Geometry: final body of the model. Coordinates: model frame, mm. A direction names the side the tool comes from. Round coordinates to 2 decimals unless told otherwise and drop trailing zeros. Order: outer loops, then holes, each group sorted by start corner. A loop starts at its lowest first (then second) coordinate and runs counter-clockwise, first axis right, second up. Notation, with made-up numbers: (42.5, -34.5) -> (82.5, -34.5) arc R22 cw to (82.5, -12.5) -> close; hole circle Ø1 at (36.25, 54.25). An arc over 180 degrees is marked (long way). Put each result on its own line as item: value.
```python
from build123d import *

# Parameters (mm, degrees)
SKETCH1_W           = 75
SKETCH1_H           = 75
BOSS_EXTRUDE1_DEPTH = 50
SKETCH2_W           = 71
SKETCH2_H           = 71
CUT_EXTRUDE1_DEPTH  = 48
CUT_EXTRUDE6_DEPTH  = 2
FILLET4_R           = 5
FILLET5_R           = 5
FILLET6_R           = 5
FILLET7_R           = 5
SKETCH4_W           = 10
SKETCH4_H           = 10
BOSS_EXTRUDE2_DEPTH = 44
SKETCH5_W           = 10
SKETCH5_H           = 10
BOSS_EXTRUDE3_DEPTH = 44
SKETCH8_W           = 51
SKETCH8_H           = 1
BOSS_EXTRUDE4_DEPTH = 10
SKETCH9_W           = 51
SKETCH9_H           = 1
BOSS_EXTRUDE5_DEPTH = 10
SKETCH11_R          = 3.25
CUT_EXTRUDE8_DEPTH  = 2.5
SKETCH12_R          = 4.375
CUT_EXTRUDE9_DEPTH  = 2
SKETCH13_R          = 5.838
CUT_EXTRUDE10_DEPTH = 2


with BuildPart() as part:
    # Sketch1 → Boss-Extrude1 (new body)
    with BuildSketch(Plane(origin=(0, 0, 0), x_dir=(1, 0, 0), z_dir=(0, 1, 0))):
        Rectangle(SKETCH1_W, SKETCH1_H)
    extrude(amount=BOSS_EXTRUDE1_DEPTH)

    # Sketch2 → Cut-Extrude1 (cut)
    with BuildSketch(Plane(origin=(0, 50, 0), x_dir=(1, 0, 0), z_dir=(0, 1, 0))):
        Rectangle(SKETCH2_W, SKETCH2_H)
    extrude(amount=-CUT_EXTRUDE1_DEPTH, mode=Mode.SUBTRACT)

    # Sketch3 → Cut-Extrude6 (cut)
    with BuildSketch(Plane.XZ):
        with BuildLine():
            add(Edge.make_bspline(
                [(8.333333333, 0), (8.451740367, 0.002755681), (8.687804992, 0.024362572), (9.156850661, 0.091751534), (10.280456566, 0.34563371), (11.894311549, 0.927153054), (13.898826649, 2.013834871), (16.012913856, 3.730779379), (17.760775609, 5.821518912), (19.049737677, 8.225078468), (19.814659338, 10.889902937), (19.985573746, 13.70225433), (19.539290317, 16.528302053), (18.494901563, 19.237024306), (16.925532574, 21.678165695), (14.89875072, 23.755747946), (12.484340707, 25.370708371), (9.802384445, 26.405476858), (6.98608034, 26.794959186), (4.109785684, 26.53719328), (0.722828385, 25.487699584), (-2.940307765, 23.340193971), (-6.647366, 20.112650151), (-10.3710479, 16.053559605), (-13.910491439, 11.839455496), (-17.496638537, 7.662725627), (-20.98187941, 4.115658379), (-23.987384387, 1.758333025), (-26.330229801, 0.518546697), (-27.55448652, 0.125207567), (-28.000518844, 0.031619583), (-28.254918245, 0.003498461), (-28.299650799, 0.000763354), (-28.322057313, 2.7753e-05), (-28.333267806, 1.08e-07)],
                knots=[0, 0, 0, 0, 0, 0.005562941, 0.011125882, 0.022251763, 0.05405154, 0.085851775, 0.117651832, 0.149451632, 0.181251419, 0.213051359, 0.246907992, 0.280764683, 0.314621503, 0.348478291, 0.382335072, 0.416191783, 0.450048462, 0.482370896, 0.514693479, 0.550840193, 0.615485432, 0.680130557, 0.744775838, 0.809420945, 0.874066354, 0.938711777, 0.978091789, 0.987992515, 0.997893241, 0.998946621, 0.99947331, 1, 1, 1, 1, 1], degree=4))
            add(Edge.make_bspline(
                [(8.333333333, 0), (8.451740367, -0.002755681), (8.687804992, -0.024362572), (9.156850661, -0.091751534), (10.280456566, -0.34563371), (11.894311549, -0.927153054), (13.898826649, -2.013834871), (16.012913856, -3.730779379), (17.760775609, -5.821518912), (19.049737677, -8.225078468), (19.814659338, -10.889902937), (19.985573746, -13.70225433), (19.539290317, -16.528302053), (18.494901563, -19.237024306), (16.925532574, -21.678165695), (14.89875072, -23.755747946), (12.484340707, -25.370708371), (9.802384445, -26.405476858), (6.98608034, -26.794959186), (4.109785684, -26.53719328), (0.722828385, -25.487699584), (-2.940307765, -23.340193971), (-6.647366, -20.112650151), (-10.3710479, -16.053559605), (-13.910491439, -11.839455496), (-17.496638537, -7.662725627), (-20.98187941, -4.115658379), (-23.987384387, -1.758333025), (-26.330229801, -0.518546697), (-27.55448652, -0.125207567), (-28.000518844, -0.031619583), (-28.254918245, -0.003498461), (-28.299650799, -0.000763354), (-28.322057313, -2.7753e-05), (-28.333267806, 1.08e-07)],
                knots=[0, 0, 0, 0, 0, 0.005562941, 0.011125882, 0.022251763, 0.05405154, 0.085851775, 0.117651832, 0.149451632, 0.181251419, 0.213051359, 0.246907992, 0.280764683, 0.314621503, 0.348478291, 0.382335072, 0.416191783, 0.450048462, 0.482370896, 0.514693479, 0.550840193, 0.615485432, 0.680130557, 0.744775838, 0.809420945, 0.874066354, 0.938711777, 0.978091789, 0.987992515, 0.997893241, 0.998946621, 0.99947331, 1, 1, 1, 1, 1], degree=4))
        make_face()
    extrude(amount=-CUT_EXTRUDE6_DEPTH, mode=Mode.SUBTRACT)

    # Fillet4
    fillet4_edges = [part.edges().sort_by_distance(p)[0] for p in [
        (35.5, 26, 35.5),
        (37.5, 25, 37.5),
    ]]
    fillet(fillet4_edges, radius=FILLET4_R)

    # Fillet5
    fillet5_edges = [part.edges().sort_by_distance(p)[0] for p in [
        (-35.5, 26, 35.5),
        (-37.5, 25, 37.5),
    ]]
    fillet(fillet5_edges, radius=FILLET5_R)

    # Fillet6
    fillet6_edges = [part.edges().sort_by_distance(p)[0] for p in [
        (-35.5, 26, -35.5),
        (-37.5, 25, -37.5),
    ]]
    fillet(fillet6_edges, radius=FILLET6_R)

    # Fillet7
    fillet7_edges = [part.edges().sort_by_distance(p)[0] for p in [
        (35.5, 26, -35.5),
        (37.5, 25, -37.5),
    ]]
    fillet(fillet7_edges, radius=FILLET7_R)

    # Sketch4 → Boss-Extrude2 (add)
    with BuildSketch(Plane(origin=(0, 2, 0), x_dir=(1, 0, 0), z_dir=(0, 1, 0))):
        with Locations((30.5, 30.5)):
            Rectangle(SKETCH4_W, SKETCH4_H)
    extrude(amount=BOSS_EXTRUDE2_DEPTH)

    # Sketch5 → Boss-Extrude3 (add)
    with BuildSketch(Plane(origin=(0, 2, 0), x_dir=(1, 0, 0), z_dir=(0, 1, 0))):
        with Locations((-30.5, 30.5)):
            Rectangle(SKETCH5_W, SKETCH5_H)
        with Locations((-30.5, -30.5)):
            Rectangle(SKETCH5_W, SKETCH5_H)
        with Locations((30.5, -30.5)):
            Rectangle(SKETCH5_W, SKETCH5_H)
    extrude(amount=BOSS_EXTRUDE3_DEPTH)

    # Sketch8 → Boss-Extrude4 (add)
    with BuildSketch(Plane(origin=(-35.5, 0, 0), x_dir=(0, 0, -1), z_dir=(1, 0, 0))):
        with Locations((0, 24.5)):
            Rectangle(SKETCH8_W, SKETCH8_H)
    extrude(amount=BOSS_EXTRUDE4_DEPTH)

    # Sketch9 → Boss-Extrude5 (add)
    with BuildSketch(Plane(origin=(-35.5, 0, 0), x_dir=(0, 0, -1), z_dir=(1, 0, 0))):
        with Locations((0, 27.11)):
            Rectangle(SKETCH9_W, SKETCH9_H)
    extrude(amount=BOSS_EXTRUDE5_DEPTH)

    # Sketch11 → Cut-Extrude8 (cut)
    with BuildSketch(Plane(origin=(0, 46, 0), x_dir=(1, 0, 0), z_dir=(0, 1, 0))):
        with Locations(Location((30.5, 30.5, 0), (0, 0, 270))):
            Circle(SKETCH11_R)
        with Locations(Location((-30.5, 30.5, 0), (0, 0, 270))):
            Circle(SKETCH11_R)
        with Locations(Location((-30.5, -30.5, 0), (0, 0, 270))):
            Circle(SKETCH11_R)
    extrude(amount=-CUT_EXTRUDE8_DEPTH, mode=Mode.SUBTRACT)

    # Sketch12 → Cut-Extrude9 (cut)
    with BuildSketch(Plane(origin=(0, 0, 35.5), x_dir=(-1, 0, 0), z_dir=(0, 0, -1))):
        with Locations((17.5, 35)):
            Circle(SKETCH12_R)
    extrude(amount=-CUT_EXTRUDE9_DEPTH, mode=Mode.SUBTRACT)

    # Sketch13 → Cut-Extrude10 (cut)
    with BuildSketch(Plane(origin=(0, 0, 35.5), x_dir=(-1, 0, 0), z_dir=(0, 0, -1))):
        with Locations((17.5, 15)):
            Circle(SKETCH13_R)
    extrude(amount=-CUT_EXTRUDE10_DEPTH, mode=Mode.SUBTRACT)


solid = part.part
```
1. Cut plane A-A on y = 35. Return loops of the section in (x, z) (3 decimals), and give its area (3 significant figures).
Ans:
outline: (-37.5, -32.5) arc R5 ccw to (-32.5, -37.5) -> (32.5, -37.5) arc R5 ccw to (37.5, -32.5) -> (37.5, 32.5) arc R5 ccw to (32.5, 37.5) -> (-13.125, 37.5) -> (-13.125, 35.5) -> (25.5, 35.5) -> (25.5, 25.5) -> (35.5, 25.5) -> (35.5, -25.5) -> (25.5, -25.5) -> (25.5, -35.5) -> (-25.5, -35.5) -> (-25.5, -25.5) -> (-35.5, -25.5) -> (-35.5, 25.5) -> (-25.5, 25.5) -> (-25.5, 35.5) -> (-21.875, 35.5) -> (-21.875, 37.5) -> (-32.5, 37.5) arc R5 ccw to (-37.5, 32.5) -> close
area: 945 mm²
2. Contact query for flat-ended pins moving along their axis: P1, Ø4, axis at x = 13, z = -4, coming from the -Y side; P2, Ø3, axis at x = -31, z = 12.5, coming from the +Y side; P3, Ø7.5, axis at x = 30.5, z = -30.5, coming from the +Y side; P4, Ø5, axis at x = -30.5, z = -31, coming from the +Y side. Output: stop coordinate, or through.
Ans:
P1: through
P2: y = 27.61
P3: y = 46
P4: y = 43.5
3. Cut plane C-C on y = 15. Return loops of the section in (x, z).
Ans:
outline: (-37.5, -32.5) arc R5 ccw to (-32.5, -37.5) -> (32.5, -37.5) arc R5 ccw to (37.5, -32.5) -> (37.5, 32.5) arc R5 ccw to (32.5, 37.5) -> (-11.66, 37.5) -> (-11.66, 35.5) -> (25.5, 35.5) -> (25.5, 25.5) -> (35.5, 25.5) -> (35.5, -25.5) -> (25.5, -25.5) -> (25.5, -35.5) -> (-25.5, -35.5) -> (-25.5, -25.5) -> (-35.5, -25.5) -> (-35.5, 25.5) -> (-25.5, 25.5) -> (-25.5, 35.5) -> (-23.34, 35.5) -> (-23.34, 37.5) -> (-32.5, 37.5) arc R5 ccw to (-37.5, 32.5) -> close
4. Set-up query: faces 5 (the face through (-13.2, 18.95, 36.49)), 6 (the face through (15, 2, 0)), 7 (the face through (0, 26, -35.5)). Return all of +Z, -Z, +X, -X, +Y, -Y with unobstructed straight access to the full face (end or side cutting, diameter ignored); none if empty.
Ans:
face 5: +Z
face 6: none
face 7: +Y
5. Cut plane B-B on x = 16.5. State how many separate pieces and enclosed holes the cut face has, and give its area (3 significant figures).
Ans:
separate pieces: 3
enclosed holes: 0
area: 272 mm²
6. Material intervals for probe 1 along X at (y, z) = (45.05, 30.5); probe 2 along Y at (x, z) = (-17.5, 36.15) (3 decimals); probe 3 along X at (y, z) = (45, -30.5), sorted ascending.
Ans:
probe 1: -37.5 to -33.75, -27.25 to -25.5, 25.5 to 37.5
probe 2: 0 to 9.162, 20.838 to 30.625, 39.375 to 50
probe 3: -37.5 to -33.75, -27.25 to -25.5, 25.5 to 27.25, 33.75 to 37.5
7. Draft query along Y for faces 1 (the face through (0, 50, 36)), 2 (the face through (-35.5, 13, 0)), 3 (the face through (37.5, 25, 0)), 4 (the face through (-31, 24, 0)). Return one class per face: +Y half, -Y half, draft (parallel to the pull), parting line (faces both ways), or undercut.
Ans:
face 1: +Y half
face 2: undercut
face 3: draft
face 4: undercut
